Here's how the part is built. I have some questions about the finished solid (model axes, mm). A direction names the side the tool comes from. Round coordinates to 2 decimals unless told otherwise and drop trailing zeros. Order: outer loops, then holes, each group sorted by start corner. A loop starts at its lowest first (then second) coordinate and runs counter-clockwise, first axis right, second up.
Autodesk Inventor part; units mm, degrees
ref_plane "YZ Plane" through (0, 0, 0) normal (1, 0, 0) x (0, 1, 0)
ref_plane "XZ Plane" through (0, 0, 0) normal (0, 1, 0) x (-1, 0, 0)
ref_plane "XY Plane" through (0, 0, 0) normal (0, 0, 1) x (1, 0, 0)
sketch "Sketch1" plane through (0, 0, 0) normal (1, 0, 0) x (0, 1, 0)
  line L0 (0, 0) -> (33.25, 0)
  line L1 (33.25, 0) -> (33.25, -33.25)
  line L2 (33.25, -33.25) -> (0, -33.25)
  line L3 (0, -33.25) -> (0, 0)
  dimension "d0" = 33.25
  dimension "d1" = 33.25
extrude "Extrusion1" add sketch "Sketch1" along normal blind 30
sketch "Sketch2" plane through (30, 0, 0) normal (1, 0, 0) x (0, 0, -1)
  line L0 (3.25, 3.25) -> (30, 3.25)
  line L1 (30, 3.25) -> (30, 30)
  line L2 (30, 30) -> (3.25, 30)
  line L3 (3.25, 30) -> (3.25, 3.25)
  point P0 (0, 0)
  dimension "d4" = 26.75
  dimension "d5" = 26.75
sketch "Sketch3" plane through (30, 0, 0) normal (1, 0, 0) x (0, 0, -1)
  line L0 (33.25, 0) -> (33.25, 33.25)
  line L1 (0, 0) -> (33.25, 0)
  line L2 (33.25, 0) -> (33.25, 33.25)
  line L3 (33.25, 33.25) -> (0, 33.25)
  line L4 (0, 33.25) -> (0, 0)
sketch "Sketch4" plane through (30, 0, 0) normal (1, 0, 0) x (0, 0, -1)
  line L0 (3.25, 3.25) -> (30, 3.25)
  line L1 (30, 3.25) -> (30, 30)
  line L2 (30, 30) -> (3.25, 30)
  line L3 (3.25, 30) -> (3.25, 3.25)
  line L4 (0, 33.25) -> (0, 0)
  line L5 (33.25, 0) -> (33.25, 33.25)
  line L6 (0, 0) -> (33.25, 0)
  line L7 (33.25, 0) -> (33.25, 33.25)
  line L8 (33.25, 33.25) -> (0, 33.25)
  line L9 (0, 33.25) -> (0, 0)
  dimension "d6" = 26.75
  dimension "d7" = 26.75
extrude "Extrusion2" cut sketch "Sketch4" against normal blind 3
chamfer "Chamfer1" distance 1.875 angle 45 8 edges at (13.5, 33.25, 0) (13.5, 33.25, -33.25) (28.5, 30, -3.25) (28.5, 30, -30) (28.5, 3.25, -3.25) (13.5, 0, 0) (28.5, 3.25, -30) (13.5, 0, -33.25)
sketch "Sketch5" plane through (30, 0, 0) normal (1, 0, 0) x (0, 0, -1)
  line L0 (9.875, 9.875) -> (23.375, 9.875)
  line L1 (23.375, 9.875) -> (23.375, 23.375)
  line L2 (23.375, 23.375) -> (9.875, 23.375)
  line L3 (9.875, 23.375) -> (9.875, 9.875)
  line L4 (28.125, 30) -> (5.125, 30)
  line L5 (30, 5.125) -> (30, 28.125)
  line L6 (3.25, 3.25) -> (30, 3.25)
  line L7 (30, 3.25) -> (30, 30)
  line L8 (30, 30) -> (3.25, 30)
  line L9 (3.25, 30) -> (3.25, 3.25)
  point P0 (0, 0)
  dimension "d13" = 13.5
  dimension "d14" = 13.5
  dimension "d15" = 6.625
  dimension "d16" = 6.625
extrude "Extrusion3" cut sketch "Sketch5" against normal blind 26.75 contours L3 L2 L1 L0
sketch "Sketch6" plane through (0, 1.875, 0) normal (0, 0, 1) x (1, 0, 0)
  point P0 (0, -1.875)
sketch "Sketch7" plane through (0, 1.875, 0) normal (0, 0, 1) x (1, 0, 0)
  circle A0 centre (18.125, 14.75) radius 4.625
  point P0 (0, -1.875)
  dimension "d19" = 9.25
extrude "Extrusion4" cut sketch "Sketch7" against normal blind 33.25
sketch "Sketch8" plane through (0, 0, -31.375) normal (0, -1, 0) x (1, 0, 0)
  circle A0 centre (18.125, 14.75) radius 4.625
  point P0 (0, 31.375)
  dimension "d22" = 9.25
extrude "Extrusion5" cut sketch "Sketch8" against normal blind 33.25
thread "Thread1"
thread "Thread2"
thread "Thread3"
thread "Thread4"
properties part number "cuvette holder blockBASE"
1) If we section it at C-C (y = 4.5): Write out the boundary of the cut face in (x, z) (3 decimals), plus the area to 3 significant figures.
2) I'm going to push flat-ended pins straight in: pin 1 (0.9 mm diameter, centred on x = 28, y = 17.5, fed in from -Z); pin 2 (1.5 mm diameter, centred on x = 15.5, y = 18.5, fed in from -Z) (3 decimals); pin 3 (4 mm diameter, centred on y = 14, z = -15, fed in from +X); pin 4 (0.9 mm diameter, centred on x = 29, z = -18.5, fed in from -Y). Where does each tip first touch, or does it pass through?
3) For faces 1 (the flat face through (29, 17, -3.25)), 2 (the flat face through (14, 23.375, -20)), 3 (the flat face through (28.521, 29.076, -29.049)), 4 (the flat face through (29, 3.25, -16)), which set-ups out of +Z, -Z, +X, -X, +Y, -Y let a thin tool reach every point of the face, with its end or its side?
4) I need wall thicknesses on line 1 (Y direction, x = 26.75, z = -14) (3 decimals); line 2 (Z direction, x = 28.5, y = 10) (3 decimals); line 3 (Z direction, x = 7.75, y = 12) (3 decimals). Which ranges of each line are inside material? Lowest first, please.
5) If we section it at A-A (x = 24): Write out the boundary of the cut face in (y, z) (3 decimals).
6) We'd pull the mould along X, two halves only. Please class faces 5 (the flat face through (28.521, 29.049, -4.174)), 6 (the flat face through (0, 16, -16)), 7 (the cylindrical face through (13.504, 16.828, -28.243)), 8 (the flat face through (27, 17, -2)): +X half, -X half, draft (parallel to the pull), parting line (faces both ways), or undercut.
7) If we section it at B-B (z = -20): Write out the boundary of the cut face in (x, y) (3 decimals).
8) If we section it at D-D (x = 18.25): Write out the boundary of the cut face in (y, z) (3 decimals).
Solutions:
1. outline: (0, -33.25) - (27, -33.25) - (27, -29.375) - (30, -29.375) - (30, -3.875) - (27, -3.875) - (27, 0) - (0, 0) - close; hole circle Ø9.25 at (18.125, -16.625)
1. area: 907 mm2
2. pin 1: stops at z = -30
2. pin 2: passes through
2. pin 3: stops at x = 3.25
2. pin 4: stops at y = 3.25
3. face 1: +Z, +X, +Y, -Y
3. face 2: +X
3. face 3: -Z, +X, +Y
3. face 4: +Z, -Z, +X, -Y
4. line 1: y = 0 to 9.875, 23.375 to 33.25
4. line 2: z = -30 to -23.375, -9.875 to -3.25
4. line 3: z = -33.25 to -23.375, -9.875 to 0
5. outline: (0, -31.375) - (1.875, -33.25) - (31.375, -33.25) - (33.25, -31.375) - (33.25, -1.875) - (31.375, 0) - (1.875, 0) - (0, -1.875) - close; hole (9.875, -23.375) - (23.375, -23.375) - (23.375, -9.875) - (9.875, -9.875) - close
6. face 5: draft
6. face 6: -X half
6. face 7: undercut
6. face 8: +X half
7. outline: (0, 0) - (14.963, 0) - (14.963, 9.875) - (3.25, 9.875) - (3.25, 23.375) - (14.963, 23.375) - (14.963, 33.25) - (0, 33.25) - close; (21.287, 0) - (27, 0) - (27, 3.25) - (30, 3.25) - (30, 9.875) - (21.287, 9.875) - close; (21.287, 23.375) - (30, 23.375) - (30, 30) - (27, 30) - (27, 33.25) - (21.287, 33.25) - close
8. outline: (0, -31.375) - (1.875, -33.25) - (12.002, -33.25) - (12.002, -23.375) - (9.875, -23.375) - (9.875, -21.248) - (0, -21.248) - close; (0, -12.002) - (9.875, -12.002) - (9.875, -9.875) - (12.002, -9.875) - (12.002, 0) - (1.875, 0) - (0, -1.875) - close; (21.248, -33.25) - (31.375, -33.25) - (33.25, -31.375) - (33.25, -21.248) - (23.375, -21.248) - (23.375, -23.375) - (21.248, -23.375) - close; (21.248, -9.875) - (23.375, -9.875) - (23.375, -12.002) - (33.25, -12.002) - (33.25, -1.875) - (31.375, 0) - (21.248, 0) - close
